Could you check a few things on this model? Use its own coordinates, in mm. A direction names the side the tool comes from. Give positions to 0.01 mm unless a question says otherwise; leave off trailing zeros. Write each loop counter-clockwise with the first axis right and the second up, starting at its lowest first coordinate (ties: lowest second). Pieces come first, ordered by that corner, then holes. Notation, with made-up numbers: (56.5, -2) - (79.5, -2) arc R21 cw to (79.5, 23) - close; hole circle Ø1 at (34, 27). An arc over 180 degrees is marked (long way). Use one line per item in the form item = value.
```python
from build123d import *

# Parameters (mm, degrees)
SKETCH2_R           = 47.5
BOSS_EXTRUDE1_DEPTH = 13
SKETCH2_4_R         = 42.5
SKETCH2_4_R_2       = 5
CUT_EXTRUDE1_DEPTH  = 8
CUT_EXTRUDE2_DEPTH  = 9
FILLET1_R           = 3
FILLET2_R           = 3
CUT_EXTRUDE4_DEPTH  = 5
CIRPATTERN1_COUNT   = 8


# Read off the part's stored shape, not the designer's step: CBORE for M3 Hex Head Machine Screw1
with BuildPart() as part:
    # Sketch2 → Boss-Extrude1 (new body)
    with BuildSketch(Plane(origin=(0, 0, 0), x_dir=(0, 0, -1), z_dir=(1, 0, 0))):
        with Locations(Location((0, 0, 0), (0, 0, 180))):
            Circle(SKETCH2_R)
    extrude(amount=BOSS_EXTRUDE1_DEPTH)

    # Sketch2<4> → Cut-Extrude1 (cut)
    with BuildSketch(Plane(origin=(0, 0, 0), x_dir=(0, 0, -1), z_dir=(1, 0, 0))):
        Circle(SKETCH2_4_R)
        Circle(SKETCH2_4_R_2, mode=Mode.SUBTRACT)
    extrude(amount=CUT_EXTRUDE1_DEPTH, mode=Mode.SUBTRACT)

    # Sketch2<5> → Cut-Extrude2 (cut)
    with BuildSketch(Plane(origin=(0, 0, 0), x_dir=(0, 0, -1), z_dir=(1, 0, 0))):
        with BuildLine():
            ThreePointArc((1.375, 1.452368755), (0, 2), (-1.375, 1.452368755))
            Line((-1.375, 1.452368755), (-1.375, -1.452368755))
            ThreePointArc((-1.375, -1.452368755), (0, -2), (1.375, -1.452368755))
            Line((1.375, -1.452368755), (1.375, 1.452368755))
        make_face()
    extrude(amount=CUT_EXTRUDE2_DEPTH, mode=Mode.SUBTRACT)

    # Fillet1
    fillet1_edges = [part.edges().sort_by_distance(p)[0] for p in [
        (8, 0, 5),
    ]]
    fillet(fillet1_edges, radius=FILLET1_R)

    # Fillet2
    fillet2_edges = [part.edges().sort_by_distance(p)[0] for p in [
        (8, 0, 42.5),
    ]]
    fillet(fillet2_edges, radius=FILLET2_R)

    # Sketch4 → Cut-Extrude4 (cut)
    with BuildSketch(Plane(origin=(13, 0, 0), x_dir=(0, 0, -1), z_dir=(1, 0, 0))):
        Polygon((0, 8), (6.83592916, 24.25), (0, 40.5), (-6.83592916, 24.25), align=None)
    cut_extrude4 = extrude(amount=-CUT_EXTRUDE4_DEPTH, mode=Mode.SUBTRACT)

    # CirPattern1: Cut-Extrude4 ×8 about axis
    cirpattern1_axis = Axis((0, -0.784667472, 0), (1, 0, 0))
    for i in range(1, CIRPATTERN1_COUNT):
        add(cut_extrude4.rotate(cirpattern1_axis, i * 360 / CIRPATTERN1_COUNT), mode=Mode.SUBTRACT)

    # CBORE for M3 Hex Head Machine Screw1 out → CBORE for M3 Hex Head Machine Screw1 (revolve, cut)
    with BuildSketch(Plane.YX):
        Polygon((0, 9), (1.7, 9), (1.7, 10.7), (4.2, 10.7), (4.2, 12.975), (4.225, 13), (0, 13), align=None)
    revolve(axis=Axis((0, 0, 0), (1, 0, 0)), mode=Mode.SUBTRACT)


solid = part.part
```
1. If we mould it in two halves opening along Z, with no side actions, what happens to faces 3 (the face through (10.54, 32.49, 3.37)), 4 (the face through (0, 0, 2))? For each: pulls with the +Z half, pulls with the -Z half, needs draft (parallel to the pull), parting line crosses it, or undercut.
Response values:
face_3 = undercut
face_4 = needs draft
2. If I drill on line 1 (Y direction, x = 2.7, z = 0); line 2 (Z direction, x = 10.5, y = -21); line 3 (Z direction, x = 11, y = -26.5), over which ranges is the centre line in solid material (lowest first)? Write a range as from..to.
Response values:
line_1 = -47.5..-42.5, -5..-2, 2..5, 42.5..47.5
line_2 = -42.61..-25.53, -11.92..-4.81, 4.81..11.92, 25.53..42.61
line_3 = -39.42..-27.77, -20.67..-6.55, 6.55..20.67, 27.77..39.42
3. For pin 1 (3 mm diameter, centred on x = 2, z = -31, fed in from +Y); pin 2 (1.5 mm diameter, centred on x = 6, z = -18, fed in from +Y); pin 3 (6 mm diameter, centred on x = 5, y = 28.5, fed in from +Z), each with a flat end and sliding along its axis, tell me the tip position at first contact or that it passes through.
Response values:
pin_1 = 37.23
pin_2 = 44.26
pin_3 = 40.07
4. Imagine slicing it at B-B, the plane y = -21. State how many separate pieces and enclosed holes the cut face has, and give its area (3 significant figures).
Response values:
separate_pieces = 4
enclosed_holes = 0
area = 337 mm²
5. Imagine slicing it at A-A, the plane x = 2.5. List the corners of the cut face in (y, z) for me (3 decimals).
Response values:
outline = circle Ø95 at (0, 0); circle Ø10 at (0, 0); hole circle Ø85 at (0, 0); hole (-1.452, -1.375) - (1.452, -1.375) arc R2 ccw to (1.452, 1.375) - (-1.452, 1.375) arc R2 ccw to start
6. Which directions (+Z, -Z, +X, -X, +Y, -Y) give clear straight access to the entire face, cutting with the end or side of a thin tool? Please do faces 1 (the face through (10.535, 16.239, 3.466)), 2 (the face through (4, 0, -1.375)).
Response values:
face_1 = +X, -X
face_2 = -X
